```python
from build123d import *

# Parameters (mm, degrees)
BOSS_EXTRUDE1_DEPTH = 43.434
SKETCH3_W           = 3.81
SKETCH3_H           = 46.482
BOSS_EXTRUDE2_DEPTH = 43.688
BOSS_EXTRUDE5_DEPTH = 39.624
SKETCH9_R           = 6.35
CUT_EXTRUDE1_DEPTH  = 44.434
SKETCH10_R          = 1.5875
CUT_EXTRUDE2_DEPTH  = 4.81
SKETCH12_W          = 45.72
SKETCH12_H          = 43.434
BOSS_EXTRUDE6_DEPTH = 12.7
SKETCH13_W          = 45.72
SKETCH13_H          = 43.434
BOSS_EXTRUDE7_DEPTH = 12.7
SKETCH14_R          = 4.064
CUT_EXTRUDE3_DEPTH  = 6.35
SKETCH15_W          = 8.127430184
SKETCH15_H          = 11.729450278
BOSS_EXTRUDE8_DEPTH = 10.414


with BuildPart() as part:
    # Sketch2 → Boss-Extrude1 (new body)
    with BuildSketch(Plane.XY.offset(816.492372385)):
        with BuildLine():
            Line((35.750095932, 34.097582937), (35.750095932, 33.285263123))
            ThreePointArc((35.750095932, 33.285263123), (35.457981836, 31.445408446), (34.772439624, 29.71323416))
            ThreePointArc((34.772439624, 29.71323416), (34.62798184, 28.864383796), (35.01595222, 28.095687512))
            Line((35.01595222, 28.095687512), (38.55890274, 24.552736992))
            ThreePointArc((38.55890274, 24.552736992), (39.005633691, 24.254240914), (39.532588778, 24.14942303))
            Line((39.532588778, 24.14942303), (43.443796213, 24.14942303))
            Line((43.443796213, 24.14942303), (43.443796213, 28.31442303))
            ThreePointArc((43.443796213, 28.31442303), (43.703006711, 28.940212531), (44.328796213, 29.19942303))
            Line((44.328796213, 29.19942303), (48.113296213, 29.19942303))
            Line((48.113296213, 29.19942303), (50.653296213, 29.19942303))
            Line((50.653296213, 29.19942303), (50.653296213, 10.45042303))
            Line((50.653296213, 10.45042303), (52.685296213, 10.45042303))
            Line((52.685296213, 10.45042303), (52.685296213, 56.93242303))
            Line((52.685296213, 56.93242303), (50.653296213, 56.93242303))
            Line((50.653296213, 56.93242303), (50.653296213, 38.18342303))
            Line((50.653296213, 38.18342303), (48.113296213, 38.18342303))
            Line((48.113296213, 38.18342303), (44.328796213, 38.18342303))
            ThreePointArc((44.328796213, 38.18342303), (43.703006711, 38.442633529), (43.443796213, 39.06842303))
            Line((43.443796213, 39.06842303), (43.443796213, 43.23342303))
            Line((43.443796213, 43.23342303), (39.532588778, 43.23342303))
            ThreePointArc((39.532588778, 43.23342303), (39.005633691, 43.128605146), (38.55890274, 42.830109068))
            Line((38.55890274, 42.830109068), (35.01595222, 39.287158548))
            ThreePointArc((35.01595222, 39.287158548), (34.62798184, 38.518462264), (34.772439624, 37.6696119))
            ThreePointArc((34.772439624, 37.6696119), (35.457981836, 35.937437615), (35.750095932, 34.097582937))
        make_face()
    extrude(amount=BOSS_EXTRUDE1_DEPTH)

    # Sketch3 → Boss-Extrude2 (add)
    with BuildSketch(Plane(origin=(52.685296213, 0, 0), x_dir=(0, 0, -1), z_dir=(1, 0, 0))):
        with Locations((-858.021372385, 33.69142303)):
            Rectangle(SKETCH3_W, SKETCH3_H)
    extrude(amount=BOSS_EXTRUDE2_DEPTH)

    # Sketch8 → Boss-Extrude5 (add)
    with BuildSketch(Plane(origin=(0, 0, 856.116372385), x_dir=(-1, 0, 0), z_dir=(0, 0, -1))):
        Polygon((-96.373296213, 56.93242303), (-52.685296213, 56.93242303), (-52.685296213, 54.90042303), (-94.087296213, 54.90042303), (-94.087296213, 42.220354744), (-96.373296213, 42.220354744), (-96.373296213, 54.90042303), align=None)
        Polygon((-96.373296213, 10.45042303), (-52.685296213, 10.45042303), (-52.685296213, 12.48242303), (-94.087296213, 12.48242303), (-94.087296213, 25.69042303), (-96.373296213, 25.69042303), (-96.373296213, 12.48242303), align=None)
    extrude(amount=BOSS_EXTRUDE5_DEPTH)

    # Sketch9 → Cut-Extrude1 (cut, through all)
    with BuildSketch(Plane.XY.offset(859.926372385)):
        with Locations((73.163747061, 34.125316724)):
            Circle(SKETCH9_R)
    extrude(amount=-CUT_EXTRUDE1_DEPTH, mode=Mode.SUBTRACT)

    # Sketch10 → Cut-Extrude2 (cut, through all)
    with BuildSketch(Plane(origin=(0, 0, 856.116372385), x_dir=(-1, 0, 0), z_dir=(0, 0, -1))):
        with Locations((-89.163747266, 50.124873673)):
            Circle(SKETCH10_R)
        with Locations((-57.921747266, 50.14642303)):
            Circle(SKETCH10_R)
        with Locations((-57.163746856, 18.90442303)):
            Circle(SKETCH10_R)
        with Locations((-88.405746856, 18.882873673)):
            Circle(SKETCH10_R)
    extrude(amount=-CUT_EXTRUDE2_DEPTH, mode=Mode.SUBTRACT)

    # Sketch12 → Boss-Extrude6 (add)
    with BuildSketch(Plane(origin=(0, 56.93242303, 0), x_dir=(1, 0, 0), z_dir=(0, 1, 0))):
        with Locations((73.513296213, -838.209372385)):
            Rectangle(SKETCH12_W, SKETCH12_H)
    extrude(amount=BOSS_EXTRUDE6_DEPTH)

    # Sketch13 → Boss-Extrude7 (add)
    with BuildSketch(Plane.XZ.offset(-10.45042303)):
        with Locations((73.513296213, 838.209372385)):
            Rectangle(SKETCH13_W, SKETCH13_H)
    extrude(amount=BOSS_EXTRUDE7_DEPTH)

    # Sketch14 → Cut-Extrude3 (cut)
    with BuildSketch(Plane.XY.offset(859.926372385)):
        with Locations((73.163747061, 63.28242303)):
            Circle(SKETCH14_R)
        with Locations((73.163747061, 4.10042303)):
            Circle(SKETCH14_R)
    extrude(amount=-CUT_EXTRUDE3_DEPTH, mode=Mode.SUBTRACT)

    # Sketch15 → Boss-Extrude8 (add)
    with BuildSketch(Plane.XY.offset(859.926372385)):
        with Locations((92.309581121, 53.763579533)):
            Rectangle(SKETCH15_W, SKETCH15_H)
    extrude(amount=BOSS_EXTRUDE8_DEPTH)


solid = part.part
```
The model under review builds one solid part; all positions refer to its coordinate system, in mm. A direction names the side the tool comes from. Round coordinates to 2 decimals unless told otherwise and drop trailing zeros. Loops run counter-clockwise (first coordinate to the right, second up) from the corner with the lowest first, then second, coordinate; pieces in that order, holes last. Notation, with made-up numbers: M 27,-22.75 L 83,-22.75 A26 ccw 83,3.25 Z; hole C 8.5,65.5 d6. An arc over 180 degrees is marked long. Write item = value, one per line.
Item 1: Take a section at D-D on z = 855. State how many separate pieces and enclosed holes the cut face has, then the cut area to 3 significant figures.
Return value:
separate_pieces = 1
enclosed_holes = 2
area = 1,600 mm2
Item 2: For line 1 (Y direction, x = 84, z = 840.5); line 2 (Y direction, x = 74, z = 856); line 3 (X direction, y = 23, z = 832.5), list the stretches that pass through material, from the lowest coordinate up. Write a range as [from, to].
Return value:
line_1 = [-2.25, 12.48], [54.9, 69.63]
line_2 = [-2.25, 0.12], [8.08, 12.48], [54.9, 59.31], [67.26, 69.63]
line_3 = [50.65, 52.69], [94.09, 96.37]
Item 3: Take a section at A-A on y = 45. Write out the cut boundary in (x, z).
Return value:
outline = M 50.65,816.49 L 52.69,816.49 L 52.69,856.12 L 94.09,856.12 L 94.09,816.49 L 96.37,816.49 L 96.37,859.93 L 50.65,859.93 Z
Item 4: Take a section at C-C on x = 65.5. Write out the cut boundary in (y, z), then the cut area to 3 significant figures.
Return value:
outline = M -2.25,816.49 L 12.48,816.49 L 12.48,856.12 L 54.9,856.12 L 54.9,816.49 L 69.63,816.49 L 69.63,859.93 L -2.25,859.93 Z
area = 1,440 mm2
Item 5: Insertion check: P1, Ø4, axis at x = 57.92, y = 50.15, coming from the -Z side; P2, Ø1.5, axis at y = 52, z = 849, coming from the -X side; P3, Ø5, axis at y = 51, z = 863.5, coming from the -X side; P4, Ø4.5, axis at y = 26, z = 834, coming from the +X side. Each pin has a flat end and moves straight along its axis. Give the tip position at first contact, or say it passes through.
Return value:
P1 = 856.12
P2 = 50.65
P3 = 88.25
P4 = 96.37
Item 6: Machinability: for faces 1 (the flat face through (50.653, 54, 839)), 2 (the cylindrical face through (57.37, 20.48, 857.99)), 3 (the flat face through (73, 54.9, 837)), 4 (the cylindrical face through (75.039, 59.677, 856.796)), 5 (the flat face through (95, 25.69, 837)), which of the approach directions +Z, -Z, +X, -X, +Y, -Y give a long, thin tool a straight path to every point of the face, cutting with its end or side? Answer none if there is none.
Return value:
face_1 = +Z, -Z, +Y
face_2 = +Z, -Z
face_3 = -Z
face_4 = +Z
face_5 = -Z, +X
Item 7: The part is to be moulded in two halves that separate along Y. For faces 6 (the flat face through (50.653, 14, 838)), 7 (the cylindrical face through (86.94, 18.27, 857.99)), 8 (the flat face through (92, 47.899, 865)), say which applies: released by +Y, released by -Y, zero draft, split by the parting line, or undercut.
Return value:
face_6 = zero draft
face_7 = undercut
face_8 = released by -Y
